```python
from build123d import *

# Parameters (mm, degrees)
F0_R     = 1.55
F1_DEPTH = 4


with BuildPart() as f1:
    # F0 (on Front) → F1 (new body)
    with BuildSketch(Plane.XZ):
        with BuildLine():
            Line((-14.5, 21), (-17.5, 21))
            ThreePointArc((-17.5, 21), (-19.62132, 20.12132), (-20.5, 18))
            Line((-20.5, 18), (-20.5, -18))
            ThreePointArc((-20.5, -18), (-19.62132, -20.12132), (-17.5, -21))
            Line((-17.5, -21), (17.5, -21))
            ThreePointArc((17.5, -21), (19.62132, -20.12132), (20.5, -18))
            Line((20.5, -18), (20.5, 18))
            ThreePointArc((20.5, 18), (19.62132, 20.12132), (17.5, 21))
            Line((17.5, 21), (14.5, 21))
            Line((14.5, 21), (12.94, 8))
            Line((12.94, 8), (12.94, 0))
            ThreePointArc((12.94, 0), (0, -12.882147), (-12.94, 0))
            Line((-12.94, 0), (-12.94, 8))
            Line((-12.94, 8), (-14.5, 21))
        make_face()
        with Locations((-15.95, -15.45)):
            Circle(F0_R, mode=Mode.SUBTRACT)
        with Locations((15.95, -15.45)):
            Circle(F0_R, mode=Mode.SUBTRACT)
        with Locations((-15.95, 15.45)):
            Circle(F0_R, mode=Mode.SUBTRACT)
        with Locations((15.95, 15.45)):
            Circle(F0_R, mode=Mode.SUBTRACT)
    extrude(amount=F1_DEPTH)


solid = f1.part
```
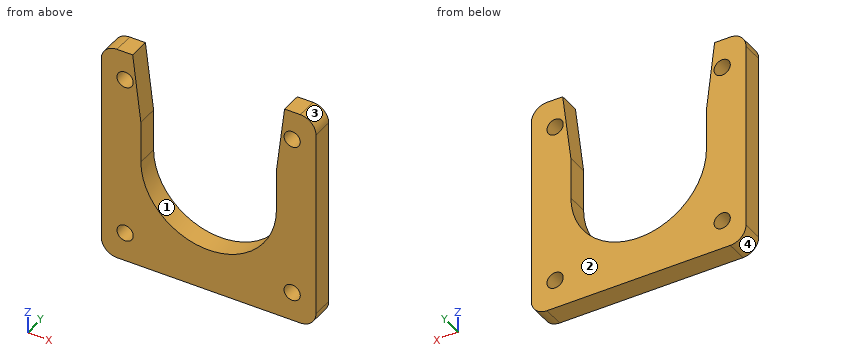
The listing builds one solid part. Answer for the finished solid, in the listing's coordinates (mm). Face numbers are marked on the shaded views. Coordinates: 2 decimals unless noted, no trailing zeros. Order: outer loops, then holes, each group sorted by start corner. A loop starts at its lowest first (then second) coordinate and runs counter-clockwise, first axis right, second up. Notation, with made-up numbers: M -24.75,2.5 L -8.75,2.5 A4 ccw -8.75,7.5 Z; hole C 28,-15 d11. An arc over 180 degrees is marked long. Answer as a JSON object with one key per item and string values. Group by question number.
1. A flat-ended cylindrical pin translates along its axis: P1, Ø5, axis at x = 15.95, z = -15.45, coming from the -Y side. Find the tip coordinate at first contact, or state that the pin passes through.
2. Section B-B on x = 15.95 is taken. Write down the section's boundary in (y, z), then the cut area to 3 significant figures.
3. Straight lines are drawn through the part: line 1 (Z direction, x = -15.95, y = -1.3); line 2 (X direction, y = -0.3, z = -16); line 3 (X direction, y = -3.3, z = -14.5). For each, find the intervals that lie inside material, in ascending order.
4. Determine the mould class of the marked faces 1, 2, 3 and 4 for opening direction X: released by +X, released by -X, zero draft, split by the parting line, or undercut.
5. Section D-D on y = -2.2 is taken. Write down the section's boundary in (x, z), then the cut area to 3 significant figures.
6. Section C-C on z = -15.45 is taken. Write down the section's boundary in (x, y), then the cut area to 3 significant figures.
7. Section A-A on z = 8.5 is taken. Write down the section's boundary in (x, y).
Values follow:
{
 "1": {"P1": "y = -4"},
 "2": {"outline": "M -4,-21 L 0,-21 L 0,-17 L -4,-17 Z; M -4,-13.9 L 0,-13.9 L 0,13.9 L -4,13.9 Z; M -4,17 L 0,17 L 0,21 L -4,21 Z", "area": "143 mm2"},
 "3": {"line 1": "-21 to -17, -13.9 to 13.9, 17 to 21", "line 2": "-20.5 to -17.4, -14.5 to 14.5, 17.4 to 20.5", "line 3": "-20.5 to -17.17, -14.73 to 14.73, 17.17 to 20.5"},
 "4": {"face 1": "undercut", "face 2": "zero draft", "face 3": "released by +X", "face 4": "released by -X"},
 "5": {"outline": "M -20.5,-18 A3 ccw -17.5,-21 L 17.5,-21 A3 ccw 20.5,-18 L 20.5,18 A3 ccw 17.5,21 L 14.5,21 L 12.94,8 L 12.94,0 A12.94 cw -12.94,0 L -12.94,8 L -14.5,21 L -17.5,21 A3 ccw -20.5,18 Z; hole C -15.95,-15.45 d3.1; hole C -15.95,15.45 d3.1; hole C 15.95,-15.45 d3.1; hole C 15.95,15.45 d3.1", "area": "859 mm2"},
 "6": {"outline": "M -20.5,-4 L -17.5,-4 L -17.5,0 L -20.5,0 Z; M -14.4,-4 L 14.4,-4 L 14.4,0 L -14.4,0 Z; M 17.5,-4 L 20.5,-4 L 20.5,0 L 17.5,0 Z", "area": "139 mm2"},
 "7": {"outline": "M -20.5,-4 L -13,-4 L -13,0 L -20.5,0 Z; M 13,-4 L 20.5,-4 L 20.5,0 L 13,0 Z"}
}
